Part model, mm, in its own coordinate system. A direction names the side the tool comes from. Coordinates: 2 decimals unless noted, no trailing zeros. Loops run counter-clockwise (first coordinate to the right, second up) from the corner with the lowest first, then second, coordinate; pieces in that order, holes last. Notation, with made-up numbers: (-16.5, 75.25) - (15.5, 75.25) arc R24 ccw to (15.5, 85.25) - close; hole circle Ø1 at (18.5, 87.25). An arc over 180 degrees is marked (long way). Use a Markdown table: item, result. Add a question column.
1) Pull direction X, two halves, no side cores. Call faces 3 (the face through (42.27, -122.47, 25.39)), 4 (the face through (-46.25, -17, 25)), 5 (the face through (-40.327, -120.168, 25.41)): +X half, -X half, draft (parallel to the pull), parting line (faces both ways), or undercut.
2) Tool access for faces 1 (the face through (0, -126.25, 25)), 2 (the face through (-43.25, -17, 25)): list every direction of +Z, -Z, +X, -X, +Y, -Y with a clear straight run to the whole face (end or side of a thin tool).
3) Drop a flat-ended pin along its axis: P1, Ø3, axis at x = 23, z = 47, coming from the +Y side. Give the stop position or say it passes through.
4) Band-saw the part on C-C (x = -10). Give the cut face in (y, z).
5) Band-saw the part on B-B (z = 15.5). Give the cut face in (x, y).
6) Band-saw the part on A-A (y = -106.5). Give the cut face in (x, z), plus the area to 3 significant figures.
7) Probe probe 1 along X at (y, z) = (15.5, 30.5); probe 2 along Y at (x, z) = (-12.5, 7.5); probe 3 along Z at (x, y) = (41.5, -43.5). List the from-to ranges inside material, lowest first. Write a range as [from, to].
from build123d import *

# Parameters (mm, degrees)
BOSS_EXTRUDE1_DEPTH = 50
BOSS_EXTRUDE2_DEPTH = 3
CHAMFER1_SIZE       = 1.5


with BuildPart() as part:
    # Sketch1 → Boss-Extrude1 (new body)
    with BuildSketch(Plane.XY):
        with BuildLine():
            Line((-46.25, 77.25220626), (-46.25, -113))
            ThreePointArc((-46.25, -113), (-42.369164851, -122.369164851), (-33, -126.25))
            Line((-33, -126.25), (33, -126.25))
            ThreePointArc((33, -126.25), (42.369164851, -122.369164851), (46.25, -113))
            Line((46.25, -113), (46.25, 77.269287137))
            ThreePointArc((46.25, 77.269287137), (46.055906569, 79.528889681), (45.479312656, 81.722292374))
            Line((45.479312656, 81.722292374), (30.588501914, 123.453005237))
            ThreePointArc((30.588501914, 123.453005237), (25.743329046, 129.829700351), (18.109189258, 132.25))
            Line((18.109189258, 132.25), (-17.946852503, 132.25))
            ThreePointArc((-17.946852503, 132.25), (-25.56302687, 129.842342367), (-30.411330997, 123.494360454))
            Line((-30.411330997, 123.494360454), (-45.464478493, 81.746566714))
            ThreePointArc((-45.464478493, 81.746566714), (-46.052142354, 79.53345153), (-46.25, 77.25220626))
        make_face()
        with BuildLine():
            ThreePointArc((-43.25, -113), (-40.247844507, -120.247844507), (-33, -123.25))
            Line((-33, -123.25), (33, -123.25))
            ThreePointArc((33, -123.25), (40.247844507, -120.247844507), (43.25, -113))
            Line((43.25, -113), (43.25, 77.269287137))
            ThreePointArc((43.25, 77.269287137), (43.099852252, 79.017281558), (42.653807903, 80.714064773))
            Line((42.653807903, 80.714064773), (27.762997162, 122.444777636))
            ThreePointArc((27.762997162, 122.444777636), (24.014844566, 127.377692725), (18.109189258, 129.25))
            Line((18.109189258, 129.25), (-17.946852503, 129.25))
            ThreePointArc((-17.946852503, 129.25), (-23.838610033, 127.387472397), (-27.589184923, 122.476769408))
            Line((-27.589184923, 122.476769408), (-42.642332419, 80.728975668))
            ThreePointArc((-42.642332419, 80.728975668), (-43.096940311, 79.016943167), (-43.25, 77.25220626))
            Line((-43.25, 77.25220626), (-43.25, -113))
        make_face(mode=Mode.SUBTRACT)
    extrude(amount=BOSS_EXTRUDE1_DEPTH)

    # Sketch3 → Boss-Extrude2 (add)
    with BuildSketch(Plane.XY.offset(50)):
        with BuildLine():
            Line((-46.25, 77.25220626), (-46.25, -113))
            ThreePointArc((-46.25, -113), (-42.369164851, -122.369164851), (-33, -126.25))
            Line((-33, -126.25), (33, -126.25))
            ThreePointArc((33, -126.25), (42.369164851, -122.369164851), (46.25, -113))
            Line((46.25, -113), (46.25, 77.269287137))
            ThreePointArc((46.25, 77.269287137), (46.055906569, 79.528889681), (45.479312656, 81.722292374))
            Line((45.479312656, 81.722292374), (30.588501914, 123.453005237))
            ThreePointArc((30.588501914, 123.453005237), (25.743329046, 129.829700351), (18.109189258, 132.25))
            Line((18.109189258, 132.25), (-17.946852503, 132.25))
            ThreePointArc((-17.946852503, 132.25), (-25.56302687, 129.842342367), (-30.411330997, 123.494360454))
            Line((-30.411330997, 123.494360454), (-45.464478493, 81.746566714))
            ThreePointArc((-45.464478493, 81.746566714), (-46.052142354, 79.53345153), (-46.25, 77.25220626))
        make_face()
    extrude(amount=BOSS_EXTRUDE2_DEPTH)

    # Chamfer1
    chamfer1_edges = [part.edges().sort_by_distance(p)[0] for p in [
        (0, -123.25, 0),
        (40.247844507, -120.247844507, 0),
        (43.25, -17.865356432, 0),
        (43.099852252, 79.017281558, 0),
        (35.208402533, 101.579421205, 0),
        (24.014844566, 127.377692725, 0),
        (0.081168378, 129.25, 0),
        (-23.838610033, 127.387472397, 0),
        (-35.115758671, 101.602872538, 0),
        (-43.096940311, 79.016943167, 0),
        (-43.25, -17.87389687, 0),
        (-40.247844507, -120.247844507, 0),
        (-46.052142354, 79.53345153, 53),
        (-46.25, -17.87389687, 53),
        (-42.369164851, -122.369164851, 53),
        (0, -126.25, 53),
        (42.369164851, -122.369164851, 53),
        (46.25, -17.865356432, 53),
        (46.055906569, 79.528889681, 53),
        (38.033907285, 102.587648806, 53),
        (25.743329046, 129.829700351, 53),
        (0.081168378, 132.25, 53),
        (-25.56302687, 129.842342367, 53),
        (-37.937904745, 102.620463584, 53),
    ]]
    chamfer(chamfer1_edges, length=CHAMFER1_SIZE)


solid = part.part
Answer block:
| question | item | result |
|---|---|---|
| 1 | face 3 | +X half |
| 1 | face 4 | -X half |
| 1 | face 5 | undercut |
| 2 | face 1 | +Z, -Z, +X, -X, -Y |
| 2 | face 2 | -Z |
| 3 | P1 | y = 131.81 |
| 4 | outline | (-126.25, 0) - (-124.75, 0) - (-123.25, 1.5) - (-123.25, 50) - (129.25, 50) - (129.25, 1.5) - (130.75, 0) - (132.25, 0) - (132.25, 51.5) - (130.75, 53) - (-124.75, 53) - (-126.25, 51.5) - close |
| 5 | outline | (-46.25, -113) arc R13.25 ccw to (-33, -126.25) - (33, -126.25) arc R13.25 ccw to (46.25, -113) - (46.25, 77.27) arc R13.25 ccw to (45.48, 81.72) - (30.59, 123.45) arc R13.25 ccw to (18.11, 132.25) - (-17.95, 132.25) arc R13.25 ccw to (-30.41, 123.49) - (-45.46, 81.75) arc R13.25 ccw to (-46.25, 77.25) - close; hole (-43.25, -113) arc R10.25 ccw to (-33, -123.25) - (33, -123.25) arc R10.25 ccw to (43.25, -113) - (43.25, 77.27) arc R10.25 ccw to (42.65, 80.71) - (27.76, 122.44) arc R10.25 ccw to (18.11, 129.25) - (-17.95, 129.25) arc R10.25 ccw to (-27.59, 122.48) - (-42.64, 80.73) arc R10.25 ccw to (-43.25, 77.25) - close |
| 6 | outline | (-46.25, 0) - (-44.75, 0) - (-43.25, 1.5) - (-43.25, 50) - (43.25, 50) - (43.25, 1.5) - (44.75, 0) - (46.25, 0) - (46.25, 51.5) - (44.75, 53) - (-44.75, 53) - (-46.25, 51.5) - close |
| 6 | area | 573 mm2 |
| 7 | probe 1 | [-46.25, -43.25], [43.25, 46.25] |
| 7 | probe 2 | [-126.25, -123.25], [129.25, 132.25] |
| 7 | probe 3 | [50, 53] |
